```python
from build123d import *

# Parameters (mm, degrees)
SKETCH1_R           = 2.4
BOSS_EXTRUDE1_DEPTH = 110
SKETCH6_R           = 1.25
BOSS_EXTRUDE2_DEPTH = 2.5
SKETCH7_R           = 1.3
CUT_EXTRUDE1_DEPTH  = 2.5
JOIN1_START         = 2
JOIN1_OUTLINE_R     = 2.4
JOIN1_DEPTH         = 10


# Read off the part's stored shape, not the designer's step: Join1
with BuildPart() as part:
    # Sketch1 → Boss-Extrude1 (new body)
    with BuildSketch(Plane.XY):
        Circle(SKETCH1_R)
    extrude(amount=BOSS_EXTRUDE1_DEPTH)

    # Sketch6 → Boss-Extrude2 (add)
    with BuildSketch(Plane(origin=(0, 0, 0), x_dir=(-1, 0, 0), z_dir=(0, 0, -1))):
        Circle(SKETCH6_R)
    extrude(amount=BOSS_EXTRUDE2_DEPTH)

    # Sketch7 → Cut-Extrude1 (cut)
    with BuildSketch(Plane.XY.offset(110)):
        Circle(SKETCH7_R)
    extrude(amount=-CUT_EXTRUDE1_DEPTH, mode=Mode.SUBTRACT)

    # Join1 outline → Join1 (add)
    with BuildSketch(Plane.XY.offset(JOIN1_START)):
        with BuildLine():
            ThreePointArc((-3.708118179, -2.272368933), (-4.244159788, -2.755671749), (-4.578357083, -3.395386049))
            ThreePointArc((-4.578357083, -3.395386049), (-4.491909089, -3.508953224), (-4.402644734, -3.620320337))
            ThreePointArc((-4.402644734, -3.620320337), (-3.701059107, -3.450910109), (-3.102375311, -3.047797308))
            ThreePointArc((-3.102375311, -3.047797308), (-2.876945397, -3.261439281), (-2.636842886, -3.458447715))
            ThreePointArc((-2.636842886, -3.458447715), (-2.962097686, -4.102754733), (-3.042635922, -4.81999654))
            ThreePointArc((-3.042635922, -4.81999654), (-2.921000374, -4.89466616), (-2.7975334, -4.966266895))
            ThreePointArc((-2.7975334, -4.966266895), (-2.204522319, -4.554854601), (-1.791887445, -3.962693577))
            ThreePointArc((-1.791887445, -3.962693577), (-1.504503928, -4.080474106), (-1.20944735, -4.177443968))
            ThreePointArc((-1.20944735, -4.177443968), (-1.279987877, -4.895737955), (-1.095989921, -5.593639789))
            ThreePointArc((-1.095989921, -5.593639789), (-0.955594371, -5.619327308), (-0.814599678, -5.64149159))
            ThreePointArc((-0.814599678, -5.64149159), (-0.410252576, -5.04364074), (-0.239395251, -4.34240612))
            ThreePointArc((-0.239395251, -4.34240612), (0.071129132, -4.348418292), (0.381290753, -4.332253266))
            ThreePointArc((0.381290753, -4.332253266), (0.574991387, -5.027524639), (0.998675593, -5.61183099))
            ThreePointArc((0.998675593, -5.61183099), (1.138869946, -5.585067166), (1.278350244, -5.554801585))
            ThreePointArc((1.278350244, -5.554801585), (1.439424051, -4.851255249), (1.345428599, -4.135652655))
            ThreePointArc((1.345428599, -4.135652655), (1.63715581, -4.029084493), (1.920533427, -3.901967754))
            ThreePointArc((1.920533427, -3.901967754), (2.352314878, -4.480316262), (2.958464434, -4.872113319))
            ThreePointArc((2.958464434, -4.872113319), (3.079523566, -4.796512755), (3.198651882, -4.717904846))
            ThreePointArc((3.198651882, -4.717904846), (3.094698483, -4.003680856), (2.748544861, -3.370356383))
            ThreePointArc((2.748544861, -3.370356383), (2.982075524, -3.165600507), (3.200397419, -2.944699876))
            ThreePointArc((3.200397419, -2.944699876), (3.81194521, -3.328016348), (4.518696259, -3.474389747))
            ThreePointArc((4.518696259, -3.474389747), (4.604270465, -3.360162718), (4.686957859, -3.243828915))
            ThreePointArc((4.686957859, -3.243828915), (4.332016737, -2.615387177), (3.78045491, -2.149874805))
            ThreePointArc((3.78045491, -2.149874805), (3.924249414, -1.874584632), (4.048030006, -1.589733962))
            ThreePointArc((4.048030006, -1.589733962), (4.756751219, -1.726249384), (5.468653116, -1.607430588))
            ThreePointArc((5.468653116, -1.607430588), (5.507185124, -1.470004087), (5.542264206, -1.331655914))
            ThreePointArc((5.542264206, -1.331655914), (4.984272126, -0.873870968), (4.301793574, -0.639040722))
            ThreePointArc((4.301793574, -0.639040722), (4.336431675, -0.330395714), (4.34895371, -0.020065668))
            ThreePointArc((4.34895371, -0.020065668), (5.059131618, 0.108657124), (5.680038067, 0.47662098))
            ThreePointArc((5.680038067, 0.47662098), (5.666323915, 0.618686743), (5.649057061, 0.760364598))
            ThreePointArc((5.649057061, 0.760364598), (4.963373946, 0.985666358), (4.24215118, 0.958099352))
            ThreePointArc((4.24215118, 0.958099352), (4.16295481, 1.258414976), (4.062527116, 1.552312606))
            ThreePointArc((4.062527116, 1.552312606), (4.678248257, 1.928888885), (5.124302402, 2.496302243))
            ThreePointArc((5.124302402, 2.496302243), (5.060194264, 2.623820499), (4.992913458, 2.749693657))
            ThreePointArc((4.992913458, 2.749693657), (4.272144611, 2.71208398), (3.609582762, 2.425842799))
            ThreePointArc((3.609582762, 2.425842799), (3.42724783, 2.67726975), (3.227433725, 2.915042461))
            ThreePointArc((3.227433725, 2.915042461), (3.665541547, 3.488613515), (3.876501304, 4.178844056))
            ThreePointArc((3.876501304, 4.178844056), (3.770657338, 4.274592757), (3.662449225, 4.367661351))
            ThreePointArc((3.662449225, 4.367661351), (3.003938474, 4.072219633), (2.48952019, 3.565962734))
            ThreePointArc((2.48952019, 3.565962734), (2.228672039, 3.734544409), (1.956457525, 3.884079679))
            ThreePointArc((1.956457525, 3.884079679), (2.15778314, 4.577181558), (2.105157224, 5.297009823))
            ThreePointArc((2.105157224, 5.297009823), (1.971872245, 5.348057577), (1.83735093, 5.395752177))
            ThreePointArc((1.83735093, 5.395752177), (1.3300338, 4.882379459), (1.033234122, 4.224479642))
            ThreePointArc((1.033234122, 4.224479642), (0.72910174, 4.287448152), (0.421250895, 4.328550414))
            ThreePointArc((0.421250895, 4.328550414), (0.358604163, 5.047575869), (0.049499995, 5.699785062))
            ThreePointArc((0.049499995, 5.699785062), (-0.093225122, 5.699237587), (-0.235891789, 5.695116774))
            ThreePointArc((-0.235891789, 5.695116774), (-0.523499308, 5.033146885), (-0.562595939, 4.312457166))
            ThreePointArc((-0.562595939, 4.312457166), (-0.868937788, 4.261308264), (-1.170848002, 4.18842643))
            ThreePointArc((-1.170848002, 4.18842643), (-1.489006294, 4.836267088), (-2.012842482, 5.332772744))
            ThreePointArc((-2.012842482, 5.332772744), (-2.14573192, 5.28070398), (-2.277276015, 5.225324292))
            ThreePointArc((-2.277276015, 5.225324292), (-2.306330934, 4.504159935), (-2.082444302, 3.818013453))
            ThreePointArc((-2.082444302, 3.818013453), (-2.349622454, 3.659655082), (-2.604817389, 3.482632247))
            ThreePointArc((-2.604817389, 3.482632247), (-3.1355182, 3.971793639), (-3.803339428, 4.245539918))
            ThreePointArc((-3.803339428, 4.245539918), (-3.908445731, 4.14898204), (-4.011101496, 4.04982281))
            ThreePointArc((-4.011101496, 4.04982281), (-3.777679787, 3.366861227), (-3.321047022, 2.807925868))
            ThreePointArc((-3.321047022, 2.807925868), (-3.512977588, 2.563745203), (-3.686991754, 2.306489282))
            ThreePointArc((-3.686991754, 2.306489282), (-4.358560998, 2.570907451), (-5.080174309, 2.584923401))
            ThreePointArc((-5.080174309, 2.584923401), (-5.14330229, 2.456917084), (-5.203205494, 2.327370316))
            ThreePointArc((-5.203205494, 2.327370316), (-4.738832052, 1.774849254), (-4.111123939, 1.418612334))
            ThreePointArc((-4.111123939, 1.418612334), (-4.201885632, 1.121587328), (-4.271217452, 0.818842159))
            ThreePointArc((-4.271217452, 0.818842159), (-4.992955982, 0.822805965), (-5.6709035, 0.575198654))
            ThreePointArc((-5.6709035, 0.575198654), (-5.683527374, 0.433031862), (-5.692587758, 0.290593566))
            ThreePointArc((-5.692587758, 0.290593566), (-5.05997879, -0.056865946), (-4.345970788, -0.162292656))
            ThreePointArc((-4.345970788, -0.162292656), (-4.323305738, -0.472047131), (-4.278591565, -0.779394136))
            ThreePointArc((-4.278591565, -0.779394136), (-4.953024594, -1.036420026), (-5.49574575, -1.512209858))
            ThreePointArc((-5.49574575, -1.512209858), (-5.456160592, -1.649336712), (-5.413154501, -1.785429457))
            ThreePointArc((-5.413154501, -1.785429457), (-4.697747354, -1.880901084), (-3.993870201, -1.721279124))
            ThreePointArc((-3.993870201, -1.721279124), (-3.860839448, -2.001929008), (-3.708118179, -2.272368933))
        make_face()
        Circle(JOIN1_OUTLINE_R, mode=Mode.SUBTRACT)
    extrude(amount=JOIN1_DEPTH)


solid = part.part
```
Build history of the part. All positions in model axes, mm. A direction names the side the tool comes from. Round coordinates to 2 decimals unless told otherwise and drop trailing zeros. Loops run counter-clockwise (first coordinate to the right, second up) from the corner with the lowest first, then second, coordinate; pieces in that order, holes last. Notation, with made-up numbers: M 50,38.5 L 90,38.5 A5 ccw 90,43.5 Z; hole C 28,14.5 d1. An arc over 180 degrees is marked long. Answer as CSV lines item,"result".
1. 3-axis set-ups, long thin cutter, end or side, ignore diameter. For faces 4 (the cylindrical face through (0.27, -1.22, -1.23)), 5 (the flat face through (2.4, -1.2, 12)), 6 (the flat face through (0, 0, -2.5)): which of +Z, -Z, +X, -X, +Y, -Y reach the whole face in a straight line?
Resolved:
face 4,"-Z"
face 5,"+Z"
face 6,"-Z, +X, -X, +Y, -Y"
2. Two-plate mould, pull along Y, no slides. Class faces 1 (the flat face through (1, -1, 0)), 2 (the cylindrical face through (1.29, 2.024, 0.986)), 3 (the cylindrical face through (-0.17, 1.29, 108.77)): released by +Y, released by -Y, zero draft, split by the parting line, or undercut.
Resolved:
face 1,"zero draft"
face 2,"split by the parting line"
face 3,"undercut"
3. Flat gauge pins, fed straight in: P1, Ø4, axis at x = -3, y = -2.5, coming from the +Z side; P2, Ø1.5, axis at y = -4, z = 49, coming from the -X side; P3, Ø3, axis at x = 2.5, z = 20, coming from the +Y side; P4, Ø6, axis at y = -2, z = 80, coming from the +X side. Where does each tip first touch, or does it go through?
Resolved:
P1,"stops at z = 110"
P2,"passes through"
P3,"stops at y = 2.18"
P4,"stops at x = 2.4"
4. Wall check: probe 1 along Y at (x, z) = (0, 109.1); probe 2 along Y at (x, z) = (-3.5, 8.5); probe 3 along Z at (x, y) = (-2.5, -3.25). Give the ranges that are in metal, low to high. Write a range as [from, to].
Resolved:
probe 1,"y = [-2.4, -1.3], [1.3, 2.4]"
probe 2,"y = [-3.35, 2.58], [2.98, 4.16]"
probe 3,"z = [2, 12]"
5. Cut at A-A on z = 52.5. Write the cut outline in (x, y), then the cut area to 3 significant figures.
Resolved:
outline,"C 0,0 d4.8"
area,"18.1 mm²"
